Model file for the job. Use its own axes, mm. Face numbers are marked on the shaded views. A direction names the side the tool comes from. Round coordinates to 2 decimals unless told otherwise and drop trailing zeros. Write each loop counter-clockwise with the first axis right and the second up, starting at its lowest first coordinate (ties: lowest second). Pieces come first, ordered by that corner, then holes. Notation, with made-up numbers: (-1.75, -8.75) - (29.25, -8.75) arc R23 cw to (29.25, 14.25) - close; hole circle Ø6 at (-6.5, 25). An arc over 180 degrees is marked (long way). One line per item, written item: value.
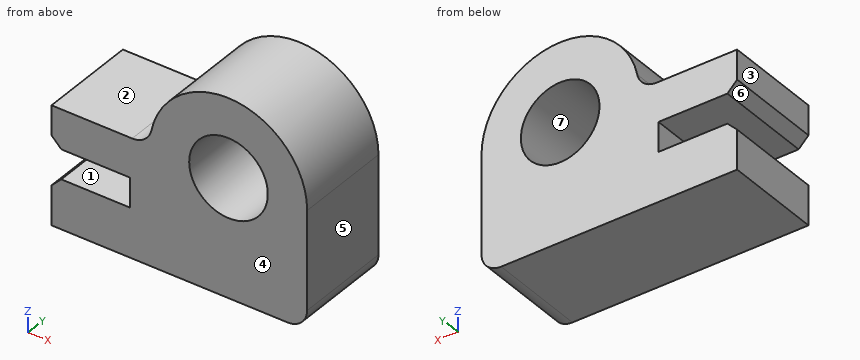
from build123d import *

# Parameters (mm, degrees)
F1_DEPTH = 50
F2_R     = 10
F3_SIZE  = 5


with BuildPart() as f1:
    # F0 (on Front) → F1 (new body)
    with BuildSketch(Plane.XZ):
        with BuildLine():
            Line((-130, 0), (0, 0))
            Line((0, 0), (0, 60))
            Line((0, 60), (-20, 60))
            ThreePointArc((-20, 60), (-40, 40), (-60, 60))
            Line((-60, 60), (-80, 60))
            Line((-80, 60), (-130, 60))
            Line((-130, 60), (-130, 40))
            Line((-130, 40), (-90, 40))
            Line((-90, 40), (-90, 25))
            Line((-90, 25), (-130, 25))
            Line((-130, 25), (-130, 0))
        make_face()
        with BuildLine():
            Line((-20, 60), (0, 60))
            ThreePointArc((0, 60), (-40, 100), (-80, 60))
            Line((-80, 60), (-60, 60))
            ThreePointArc((-60, 60), (-40, 80), (-20, 60))
        make_face()
    extrude(amount=F1_DEPTH)

    # F2
    f2_edges = [f1.edges().sort_by_distance(p)[0] for p in [
        (0, -25, 60),
        (0, -25, 0),
        (-80, -25, 60),
    ]]
    fillet(f2_edges, radius=F2_R)

    # F3
    f3_edges = [f1.edges().sort_by_distance(p)[0] for p in [
        (-130, -25, 40),
        (-130, -25, 25),
    ]]
    chamfer(f3_edges, length=F3_SIZE)


solid = f1.part
1. Band-saw the part on C-C on x = -104.5. Write the cut outline in (y, z).
Report:
outline: (-50, 0) - (0, 0) - (0, 25) - (-50, 25) - close; (-50, 40) - (0, 40) - (0, 60) - (-50, 60) - close
2. Wall check: probe 1 along Z at (x, y) = (-40, -26.5); probe 2 along Z at (x, y) = (-113.5, -31.5); probe 3 along X at (y, z) = (-31.5, 70). Give the ranges that are in metal, low to high. Write a range as [from, to].
Report:
probe 1: [0, 40], [80, 100]
probe 2: [0, 25], [40, 60]
probe 3: [-78.73, -57.32], [-22.68, -1.27]
3. Band-saw the part on A-A on x = -40. Write the cut outline in (y, z).
Report:
outline: (-50, 0) - (0, 0) - (0, 40) - (-50, 40) - close; (-50, 80) - (0, 80) - (0, 100) - (-50, 100) - close
4. Band-saw the part on D-D on z = 29. Write the cut outline in (x, y).
Report:
outline: (-90, -50) - (0, -50) - (0, 0) - (-90, 0) - close
5. Drop flat-ended pins along their axis: pin 1 (6 mm diameter, centred on x = -114.5, y = -11.5, fed in from +Z); pin 2 (7.5 mm diameter, centred on y = -27, z = 30, fed in from -X); pin 3 (5 mm diameter, centred on x = -99.5, z = 46.5, fed in from +Y). Give the stop position or say it passes through.
Report:
pin 1: z = 60
pin 2: x = -90
pin 3: y = 0
6. Mould opens along X. For the marked faces 4, 5, 6 and 7 say: released by +X, released by -X, zero draft, split by the parting line, or undercut.
Report:
face 4: zero draft
face 5: released by +X
face 6: released by -X
face 7: undercut
7. Tool access for the marked faces 1, 2 and 3: list every direction of +Z, -Z, +X, -X, +Y, -Y with a clear straight run to the whole face (end or side of a thin tool).
Report:
face 1: -X, +Y, -Y
face 2: +Z, -X, +Y, -Y
face 3: +Z, -Z, -X, +Y, -Y
8. Band-saw the part on B-B on y = -6. Write the cut outline in (x, z), plus the area to 3 significant figures.
Report:
outline: (-130, 0) - (-10, 0) arc R10 ccw to (0, 10) - (0, 60) arc R40 ccw to (-79.19, 68) arc R10 cw to (-88.99, 60) - (-130, 60) - (-130, 45) - (-125, 40) - (-90, 40) - (-90, 25) - (-125, 25) - (-130, 20) - close; hole circle Ø40 at (-40, 60)
area: 8,430 mm²
